Autodesk Inventor part; units mm, degrees
ref_plane "YZ Plane" through (0, 0, 0) normal (1, 0, 0) x (0, 1, 0)
ref_plane "XZ Plane" through (0, 0, 0) normal (0, 1, 0) x (-1, 0, 0)
ref_plane "XY Plane" through (0, 0, 0) normal (0, 0, 1) x (1, 0, 0)
sketch "草图1" plane through (0, 0, 0) normal (0, 0, 1) x (1, 0, 0)
  circle A0 centre (0, 0) radius 2.5
  dimension "d0" = 5
extrude "拉伸1" add sketch "草图1" along normal blind 2.5
sketch "草图2" plane through (0, 0, 2.5) normal (0, 0, 1) x (1, 0, 0)
  circle A0 centre (0, 0) radius 1.5
  dimension "d3" = 3
extrude "拉伸2" add sketch "草图2" along normal blind 10
thread "螺纹1"
chamfer "倒角1" distance 0.25 angle 45 1 edges at (-1.5, 0, 12.5)
sketch "草图3" plane through (0, 0, 0) normal (0, 0, -1) x (-1, 0, 0)
  line L0 (0.866, -1.5) -> (-0.866, -1.5)
  line L1 (-0.866, -1.5) -> (-1.7321, 0)
  line L2 (-1.7321, 0) -> (-0.866, 1.5)
  line L3 (-0.866, 1.5) -> (0.866, 1.5)
  line L4 (0.866, 1.5) -> (1.7321, 0)
  line L5 (1.7321, 0) -> (0.866, -1.5)
  line L6 (0, 0) -> (0, 0.2895)
  circle A0 centre (0, 0) radius 1.5
  point P0 (0, 1.5)
  dimension "d11" = 0.2895
  dimension "d12" = 1.5
extrude "拉伸3" cut sketch "草图3" against normal blind 1.25
properties part number "砂轮轴端盖螺丝"
Design review of the part built by this model. Coordinates are the model's own, in mm. A direction names the side the tool comes from. Coordinates: 2 decimals unless noted, no trailing zeros. Loops run counter-clockwise (first coordinate to the right, second up) from the corner with the lowest first, then second, coordinate; pieces in that order, holes last.
Q1. The part is to be moulded in two halves that separate along X. For faces 3 (the face through (0, 1.5, 1)), 4 (the face through (-1.5, -0.07, 7.31)), 5 (the face through (2, 0, 2.5)), 6 (the face through (1.305, 0.74, 0.616)), say which applies: +X half, -X half, draft (parallel to the pull), parting line (faces both ways), or undercut.
Reported:
face 3: undercut
face 4: parting line
face 5: draft
face 6: undercut
Q2. We need section B-B on z = 9. State the section outline as (x, y) points, and give its area (3 significant figures).
Reported:
outline: circle Ø3 at (0, 0)
area: 7.07 mm2
Q3. We need section C-C on y = 1.7. State the section outline as (x, z) points.
Reported:
outline: (-1.83, 0) - (1.83, 0) - (1.83, 2.5) - (-1.83, 2.5) - close
Q4. We need section A-A on x = 0. State the section outline as (y, z) points.
Reported:
outline: (-2.5, 0) - (-1.5, 0) - (-1.5, 1.25) - (1.5, 1.25) - (1.5, 0) - (2.5, 0) - (2.5, 2.5) - (1.5, 2.5) - (1.5, 12.25) - (1.25, 12.5) - (-1.25, 12.5) - (-1.5, 12.25) - (-1.5, 2.5) - (-2.5, 2.5) - close
Q5. Tool access review of faces 1 (the face through (0, 0, 12.5)), 2 (the face through (1.293, -0.76, 0.616)): name each direction out of +Z, -Z, +X, -X, +Y, -Y from which nothing blocks a thin tool from reaching the whole face with its end or side.
Reported:
face 1: +Z, +X, -X, +Y, -Y
face 2: -Z
Q6. To check wall thickness, follow line 1 (Z direction, x = -0.85, y = 0.2); line 2 (Z direction, x = -1.15, y = -1.8); line 3 (Y direction, x = -0.4, z = 4). State the ranges of each line that lie inside material, in increasing order.
Reported:
line 1: z = 1.25 to 12.5
line 2: z = 0 to 2.5
line 3: y = -1.45 to 1.45
Q7. For pin 1 (0.6 mm diameter, centred on x = 0.5, z = 0.5, fed in from -Y); pin 2 (1 mm diameter, centred on x = 1, z = 1.5, fed in from +Y); pin 3 (2 mm diameter, centred on x = 0.5, z = 4.5, fed in from +Y), all flat-tipped, find the tip position at first contact; note any pin that passes through.
Reported:
pin 1: stops at y = -2.49
pin 2: stops at y = 2.45
pin 3: stops at y = 1.5
